The listing builds one solid part. Answer for the finished solid, in the listing's coordinates (mm). A direction names the side the tool comes from. Coordinates: 2 decimals unless noted, no trailing zeros. Loops run counter-clockwise (first coordinate to the right, second up) from the corner with the lowest first, then second, coordinate; pieces in that order, holes last. Notation, with made-up numbers: (19.25, 76.5) - (56.25, 76.5) arc R19 cw to (56.25, 102.5) - close; hole circle Ø11 at (-13, -22). An arc over 180 degrees is marked (long way). Return JSON: item names as keys, results as strings. Group by question number.
1. Which of the six approach directions +Z, -Z, +X, -X, +Y, -Y give full straight-line access (tool end or side, diameter ignored) to faces 1 (the face through (121, 48.316, -1)), 2 (the face through (87.414, 43, -1)), 3 (the face through (88, 42.116, -2)), 4 (the face through (83, 37.116, -1))?
2. The mould has two halves that part along Z. Classify faces 5 (the face through (115.5, 43.2, -1.2)), 6 (the face through (83, 49.316, -1)), 7 (the face through (115.5, 43.2, -2.4)), 8 (the face through (101, 43, 2)): pulls with the +Z half, pulls with the -Z half, needs draft (parallel to the pull), parting line crosses it, or undercut.
3. Each of these flat-tipped pins is pushed along its axis until it touches: P1, Ø0.9, axis at y = 41.5, z = -1.5, coming from the +X side; P2, Ø0.5, axis at y = 48.5, z = -1.5, coming from the +X side; P3, Ø1, axis at x = 111.5, z = -2, coming from the +Y side; P4, Ø0.5, axis at x = 115.5, z = -2, coming from the +Y side. Where does it stop, or does it pass through?
4. Section A-A (z = -0.55) is taken. Write down the section's boundary in (x, y).
5. Find the intervals of material crossed by line 1 along X through (y, z) = (47.75, -2.55); line 2 along Y through (x, z) = (81.5, -2.4); line 3 along X through (y, z) = (37.5, -0.6), in increasing order.
Autodesk Fusion 360 part; units mm, degrees
sketch "Sketch1" plane through (0, 0, 0) normal (0, 0, 1) x (1, 0, 0)
  line L0 (82.0141, 54.0159) -> (121.4141, 54.0159)
  line L1 (121.4141, 32.4159) -> (82.0141, 32.4159)
  arc A0 (82.0141, 54.0159) -> (71.257, 42.2547) centre (82.0141, 43.2159) ccw
  arc A1 (71.257, 42.2547) -> (82.0141, 32.4159) centre (82.0141, 43.2159) ccw
  arc A2 (130.5847, 37.5114) -> (121.4141, 54.0159) centre (121.4141, 43.2159) ccw
  arc A3 (121.4141, 32.4159) -> (130.5847, 37.5114) centre (121.4141, 43.2159) ccw
  dimension "d1" = 21.6
  dimension "d58" = 39.4
extrude "Extrude1" add sketch "Sketch1" along normal blind 2
fillet "Fillet1" radius 2 4 edges at (132.2141, 43.2159, 2) (101.7141, 54.0159, 2) (71.2141, 43.2159, 2) (101.7141, 32.4159, 2)
sketch "Sketch4" plane through (0, 0, 0) normal (0, 0, -1) x (1, 0, 0)
  arc A0 (82.0141, -32.4159) -> (82.0141, -54.0159) centre (82.0141, -43.2159) ccw
  line L0 (82.0141, -54.0159) -> (121.4141, -54.0159)
  arc A1 (121.4141, -54.0159) -> (121.4141, -32.4159) centre (121.4141, -43.2159) ccw
  line L1 (121.4141, -32.4159) -> (82.0141, -32.4159)
  line L2 (71.2141, -43.2159) -> (132.2141, -43.2159) construction
  line L3 (88.4141, -37.1159) -> (88.4141, -49.3159)
  line L4 (101.7141, -32.4159) -> (101.7141, -54.0159) construction
  line L5 (72.4941, -38.1159) -> (87.4141, -38.1159)
  line L6 (87.4141, -38.1159) -> (87.4141, -48.3159)
  line L7 (87.4141, -48.3159) -> (72.4941, -48.3159)
  line L8 (77.4372, -37.1159) -> (88.4141, -37.1159)
  line L9 (88.4141, -49.3159) -> (77.4372, -49.3159)
  line L10 (77.4372, -37.1159) -> (77.4372, -49.3159)
  line L11 (115.0141, -49.3159) -> (125.991, -49.3159)
  line L12 (116.0141, -48.3159) -> (130.9341, -48.3159)
  line L13 (125.991, -37.1159) -> (125.991, -49.3159)
  line L14 (130.9341, -38.1159) -> (116.0141, -38.1159)
  line L15 (125.991, -37.1159) -> (115.0141, -37.1159)
  line L16 (116.0141, -38.1159) -> (116.0141, -48.3159)
  line L17 (115.0141, -37.1159) -> (115.0141, -49.3159)
  dimension "d18" = 17.2
  dimension "d20" = 1
  dimension "d35" = 1
  dimension "d51" = 12.2
  dimension "d52" = 1
extrude "Extrude3" add sketch "Sketch4" along normal blind 3 contours L3 L5 L6 L7 L8 L9 L10 | L11 L12 L13 L14 L15 L16 L17
sketch "Sketch6" plane through (87.4141, 0, 0) normal (-1, 0, 0) x (0, -1, 0)
  line L0 (-38.1159, 0) -> (-48.3159, 0)
  line L1 (-48.3159, 0) -> (-48.3159, -3)
  line L2 (-48.3159, -3) -> (-38.1159, -3)
  line L3 (-38.1159, -3) -> (-38.1159, 0)
  line L4 (-43.2159, -3) -> (-43.2159, 0) construction
  line L5 (-42.1159, -2.4) -> (-44.3159, -2.4)
  line L6 (-44.3159, -2.4) -> (-44.3159, -1.2)
  line L7 (-44.3159, -1.2) -> (-42.1159, -1.2)
  line L8 (-42.1159, -1.2) -> (-42.1159, -2.4)
  dimension "d23" = 2.2
  dimension "d24" = 1.2
  dimension "d25" = 0.6
extrude "Extrude4" cut sketch "Sketch6" against normal blind 33 contours L5 L6 L7 L8
The answers:
{
 "1": {"face 1": "-Z, +X", "face 2": "-Z, -X", "face 3": "+X, -X", "face 4": "-Z, +X, -X, -Y"},
 "2": {"face 5": "undercut", "face 6": "needs draft", "face 7": "undercut", "face 8": "pulls with the +Z half"},
 "3": {"P1": "stops at x = 116.01", "P2": "stops at x = 125.99", "P3": "passes through", "P4": "stops at y = 49.32"},
 "4": {"outline": "(77.44, 37.12) - (88.41, 37.12) - (88.41, 49.32) - (77.44, 49.32) - (77.44, 48.32) - (87.41, 48.32) - (87.41, 38.12) - (77.44, 38.12) - close; (115.01, 37.12) - (125.99, 37.12) - (125.99, 38.12) - (116.01, 38.12) - (116.01, 48.32) - (125.99, 48.32) - (125.99, 49.32) - (115.01, 49.32) - close"},
 "5": {"line 1": "x = 87.41 to 88.41, 115.01 to 116.01", "line 2": "y = 37.12 to 38.12, 48.32 to 49.32", "line 3": "x = 77.44 to 88.41, 115.01 to 125.99"}
}
